from build123d import *

# Parameters (mm, degrees)
BOSS_EXTRUDE1_DEPTH      = 30
BOSS_EXTRUDE1_DEPTH_BACK = 30
SKETCH1_R                = 5
SKETCH2_R                = 3
BOSS_EXTRUDE2_DEPTH      = 10


with BuildPart() as part:
    # Sketch1 → Boss-Extrude1 (new, two sides: drawn at the far end of the back side and taken through both)
    with BuildSketch(Plane(origin=(0, 0, 0), x_dir=(0, 0, -1), z_dir=(1, 0, 0)).offset(-BOSS_EXTRUDE1_DEPTH_BACK)):
        Circle(SKETCH1_R)
    extrude(amount=BOSS_EXTRUDE1_DEPTH + BOSS_EXTRUDE1_DEPTH_BACK)

    # Sketch2 → Boss-Extrude2 (add)
    with BuildSketch(Plane(origin=(30, 0, 0), x_dir=(0, 0, -1), z_dir=(1, 0, 0))):
        Circle(SKETCH2_R)
    boss_extrude2 = extrude(amount=BOSS_EXTRUDE2_DEPTH)

    # Mirror1: Boss-Extrude2 across plane
    add(boss_extrude2.mirror(Plane(origin=(0, 0, 0), x_dir=(0, 0, 1), z_dir=(1, 0, 0))))


solid = part.part
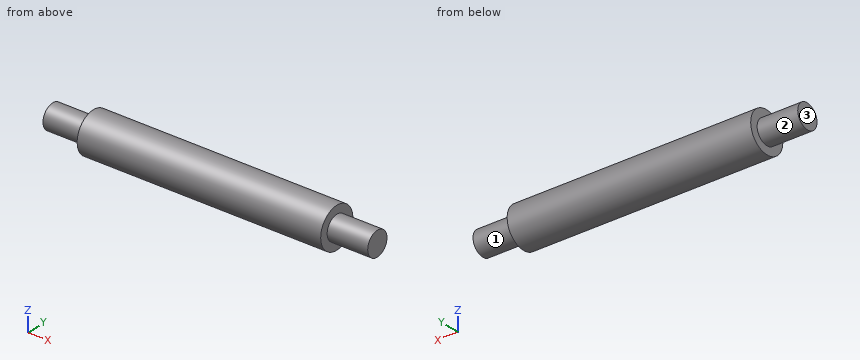
The listing builds one solid part. Answer for the finished solid, in the listing's coordinates (mm). Face numbers are marked on the shaded views. A direction names the side the tool comes from. Coordinates: 2 decimals unless noted, no trailing zeros. Order: outer loops, then holes, each group sorted by start corner. A loop starts at its lowest first (then second) coordinate and runs counter-clockwise, first axis right, second up. Notation, with made-up numbers: (-26, -25.75) -> (-6, -25.75) arc R30 cw to (-6, 2.25) -> close; hole circle Ø8 at (47.25, -28). An arc over 180 degrees is marked (long way). Answer in a Markdown table with one row per item. Add a question column.
Item 1: Which of the six approach directions +Z, -Z, +X, -X, +Y, -Y give full straight-line access (tool end or side, diameter ignored) to the marked faces 1, 2 and 3?
Item 2: Find section D-D (x = 13). Write down the section's boundary in (y, z).
Item 3: Find section C-C (x = 34). Write down the section's boundary in (y, z), then the cut area to 3 significant figures.
Item 4: Each of these flat-tipped pins is pushed along its axis until it touches: P1, Ø1, axis at y = -4, z = -3, coming from the -X side; P2, Ø2, axis at x = 18.5, y = -2, coming from the +Z side; P3, Ø6, axis at x = 11.5, y = 3.5, coming from the +Z side. Where does it stop, or does it pass through?
Item 5: Find section A-A (y = 0). Write down the section's boundary in (x, z), then the cut area to 3 significant figures.
Item 6: Find the intervals of material crossed by L1, parallel to X at y = 3.5, z = 2.5; L2, parallel to Z at x = -1, y = 4; L3, parallel to Y at x = 9, z = -1.5, in increasing order. Write a range as from..to.
Result set:
| question | item | result |
|---|---|---|
| 1 | face 1 | +X |
| 1 | face 2 | -X |
| 1 | face 3 | +Z, -Z, -X, +Y, -Y |
| 2 | outline | circle Ø10 at (0, 0) |
| 3 | outline | circle Ø6 at (0, 0) |
| 3 | area | 28.3 mm² |
| 4 | P1 | stops at x = -30 |
| 4 | P2 | stops at z = 4.9 |
| 4 | P3 | stops at z = 4.97 |
| 5 | outline | (-40, -3) -> (-30, -3) -> (-30, -5) -> (30, -5) -> (30, -3) -> (40, -3) -> (40, 3) -> (30, 3) -> (30, 5) -> (-30, 5) -> (-30, 3) -> (-40, 3) -> close |
| 5 | area | 720 mm² |
| 6 | L1 | x = -30..30 |
| 6 | L2 | z = -3..3 |
| 6 | L3 | y = -4.77..4.77 |
